Build history of the part. All positions in model axes, mm. Face numbers are marked on the shaded views. Coordinates: 2 decimals unless noted, no trailing zeros. Loops run counter-clockwise (first coordinate to the right, second up) from the corner with the lowest first, then second, coordinate; pieces in that order, holes last.
(1) Slice it at C-C (x = 1). Give the cut face in (y, z), and give its area (3 significant figures).
(2) Slice it at A-A (x = 17). Give the cut face in (y, z).
(3) Slice it at B-B (z = 23.5). Give the cut face in (x, y).
(4) Wall check: L1, parallel to X at y = -14, z = 0.6; L2, parallel to Z at x = 18, y = 42; L3, parallel to Y at x = 17, z = 0.8. Give the ranges that are in metal, low to high.
(5) Flat gauge pins, fed straight in: P1, Ø2.5, axis at x = 17, y = 40, coming from the -Z side; P2, Ø4, axis at y = -4, z = 7, coming from the +X side; P3, Ø4, axis at x = -17.3, y = -14, coming from the -Z side. Where does each tip first touch, or does it go through?
(6) Two-plate mould, pull along Z, no slides. Class the marked faces 1, 2, 3 and 4: pulls with the +Z half, pulls with the -Z half, needs draft (parallel to the pull), parting line crosses it, or undercut.
(7) Slice it at D-D (y = 7). Give the cut face in (x, z), and give its area (3 significant figures).
Autodesk Fusion 360 part; units mm, degrees
sketch "Sketch1" plane through (0, 0, 0) normal (0, 0, 1) x (1, 0, 0)
  line L0 (-25, 50) -> (25, 50)
  line L1 (25, 50) -> (25, -25)
  line L2 (25, -25) -> (-25, -25)
  line L3 (-25, -25) -> (-25, 50)
  circle A0 centre (-17.3027, -14) radius 1.5
  circle A1 centre (16.6973, -14) radius 1.5
  circle A2 centre (-17, 40) radius 1.5
  circle A3 centre (17, 39.9992) radius 1.5
  dimension "d1" = 3
  dimension "d2" = 3
  dimension "d4" = 34
  dimension "d5" = 3
  dimension "d6" = 54
  dimension "d7" = 3
  dimension "d9" = 34
  dimension "d10" = 54
extrude "Extrude1" add sketch "Sketch1" along normal blind 2 makes body 1
ref_plane "WorkPlane1" through (0, 12.5, 3) normal (0, 0, 1) x (1, 0, 0)
ref_plane "WorkPlane2" through (0, 12.5, 42) normal (0, 0, 1) x (1, 0, 0)
sketch "Sketch4" plane through (0, 0, 42) normal (0, 0, 1) x (1, 0, 0)
sketch "Sketch5" plane through (0, 0, 42) normal (0, 0, 1) x (1, 0, 0)
  line L0 (25, -25) -> (-25, -25)
  line L1 (-25, -25) -> (-25, 50)
  line L2 (-25, 50) -> (25, 50)
  line L3 (25, 50) -> (25, -25)
extrude "Extrude2" add sketch "Sketch5" against normal blind 2 separate body makes body 2
sketch "Sketch6" plane through (0, 0, 2) normal (0, 0, 1) x (-1, 0, 0)
  circle A0 centre (17, -40) radius 1.5
  circle A1 centre (-16.6973, 14) radius 1.5
  circle A2 centre (-17, -39.9992) radius 1.5
  circle A3 centre (17.3027, 14) radius 1.5
  line L0 (25, 25) -> (-25, 25)
  line L1 (-25, 25) -> (-25, -50)
  line L2 (-25, -50) -> (25, -50)
  line L3 (25, -50) -> (25, 25)
  line L4 (25, -50) -> (23, -50)
  line L5 (23, -50) -> (23, 25)
  line L6 (23, 25) -> (25, 25)
  line L7 (25, 25) -> (25, -50)
extrude "Extrude3" add sketch "Sketch6" along normal blind 39 contours L0 L2 L3 L4 L5 L6 L7 bodies 1 2
sketch "Sketch7" plane through (0, 0, 2) normal (0, 0, 1) x (-1, 0, 0)
  line L0 (23, -50) -> (23, 25)
  line L1 (23, 25) -> (-25, 25)
  line L2 (-25, 25) -> (-25, -50)
  line L3 (-25, -50) -> (23, -50)
  circle A0 centre (17.3027, 14) radius 1.5
  circle A1 centre (-17, -39.9992) radius 1.5
  circle A2 centre (-16.6973, 14) radius 1.5
  circle A3 centre (17, -40) radius 1.5
  line L4 (23, 25) -> (-25, 25)
  line L5 (-25, 25) -> (-25, 23)
  line L6 (-25, 23) -> (23, 23)
  line L7 (23, 23) -> (23, 25)
  line L8 (23, -50) -> (-25, -50)
  line L9 (-25, -50) -> (-25, -48)
  line L10 (-25, -48) -> (23, -48)
  line L11 (23, -48) -> (23, -50)
extrude "Extrude4" add sketch "Sketch7" along normal blind 38 contours L0 L2 L3 L8 L9 L10 L11 bodies 1
extrude "Extrude5" add sketch "Sketch7" along normal blind 38 contours L0 L1 L2 L4 L5 L6 L7 bodies 1
sketch "Sketch8" plane through (0, 0, 2) normal (0, 0, 1) x (-1, 0, 0)
  line L0 (23, 23) -> (-25, 23)
  line L1 (-25, 23) -> (-25, -48)
  line L2 (-25, -48) -> (23, -48)
  line L3 (23, -48) -> (23, 23)
  circle A0 centre (17, -40) radius 1.5
  circle A1 centre (-16.6973, 14) radius 1.5
  circle A2 centre (-17, -39.9992) radius 1.5
  circle A3 centre (17.3027, 14) radius 1.5
  line L4 (23, 14) -> (-25, 14)
  line L5 (-25, 14) -> (-25, 7)
  line L6 (-25, 7) -> (23, 7)
  line L7 (23, 7) -> (23, 14)
extrude "Extrude6" cut sketch "Sketch8" along normal blind 48 contours L1 L3 A1 A3 L4 L5 L6 L7 bodies 1
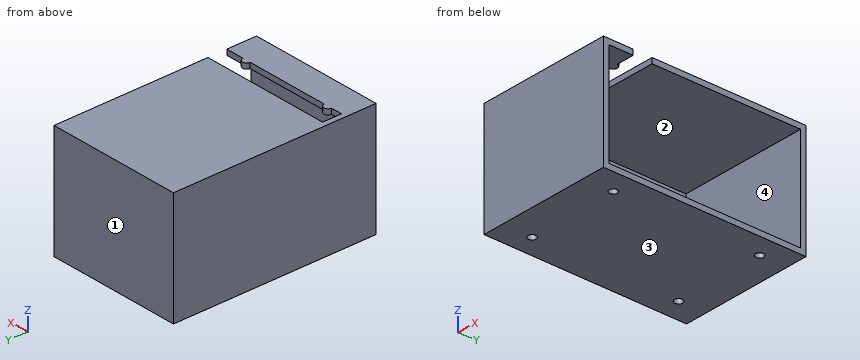
Response values:
1. outline: (-25, 0) - (50, 0) - (50, 42) - (-7, 42) - (-7, 40) - (48, 40) - (48, 2) - (-23, 2) - (-23, 40) - (-14, 40) - (-14, 42) - (-25, 42) - close
1. area: 438 mm2
2. outline: (-25, 0) - (-15.47, 0) - (-15.47, 2) - (-23, 2) - (-23, 40) - (-12.53, 40) - (-12.53, 42) - (-25, 42) - close; (-12.53, 0) - (38.5, 0) - (38.5, 2) - (-12.53, 2) - close; (-7, 40) - (48, 40) - (48, 2) - (41.5, 2) - (41.5, 0) - (50, 0) - (50, 42) - (-7, 42) - close
3. outline: (-25, -25) - (25, -25) - (25, -23) - (-23, -23) - (-23, 48) - (25, 48) - (25, 50) - (-25, 50) - close
4. L1: x = -25 to -18.8, -15.8 to 15.2, 18.2 to 25
4. L2: z = 0 to 2, 40 to 42
4. L3: y = -25 to -15.47, -12.53 to 38.5, 41.5 to 50
5. P1: stops at z = 40
5. P2: stops at x = -23
5. P3: stops at z = 0
6. face 1: needs draft
6. face 2: undercut
6. face 3: pulls with the -Z half
6. face 4: undercut
7. outline: (-25, 0) - (25, 0) - (25, 2) - (-23, 2) - (-23, 40) - (25, 40) - (25, 42) - (-25, 42) - close
7. area: 276 mm2
